Source: CAD feature listing. Evaluate the final solid. Frame: model axes, mm. Coordinates: 2 decimals unless noted, no trailing zeros. Write each loop counter-clockwise with the first axis right and the second up, starting at its lowest first coordinate (ties: lowest second). Pieces come first, ordered by that corner, then holes. Notation, with made-up numbers: M 48.5,44.25 L 55.5,44.25 A17 ccw 55.5,58.25 Z; hole C 25,-16 d7. An arc over 180 degrees is marked long. Write item = value, one per line. Start each with the question number.
1. Pin query (flat end, axial travel): pin 1 Ø3 at (x, y) = (0.9, 15.73) entering from +Z. Return the tip coordinate at first contact, or that it passes through.
2. Section query B-B (z = 0.7). Output: boundary loops of the cut face in (x, y).
3. Section query D-D (x = -33). Output: boundary loops of the cut face in (y, z), then the cut area to 3 significant figures.
4. Section query A-A (y = 0). Output: boundary loops of the cut face in (x, z).
5. Section query C-C (x = 0). Output: boundary loops of the cut face in (y, z).
6. Line query: line 1 along Y through (x, z) = (8, 2.25); line 2 along Y through (x, z) = (-12.5, 1.4); line 3 along X through (y, z) = (6, 1.65). Output: solid intervals per line, ascending.
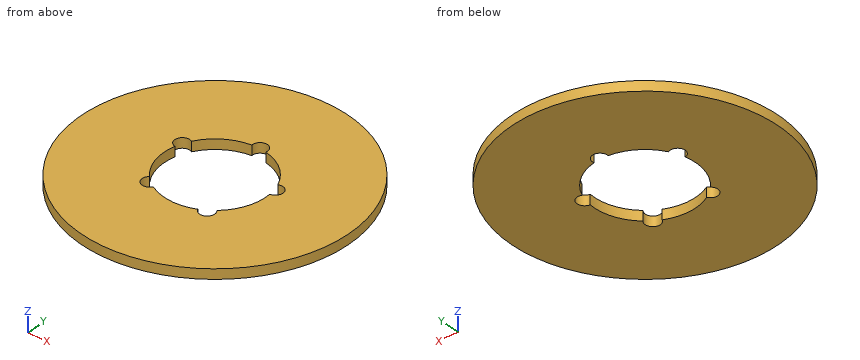
```python
from build123d import *

# Parameters (mm, degrees)
F0_R     = 40.7341209129
F1_DEPTH = 3
F2_R     = 12.35
F3_DEPTH = 5
F4_R     = 15.5
F5_DEPTH = 3
F7_R     = 2.3
F8_DEPTH = 25


# Not quite as in the source:
# - a feature names something its author has since deleted; it is built from what else it names


with BuildPart() as f1:
    # F0 (on Top) → F1 (new body)
    with BuildSketch(Plane.XY):
        Circle(F0_R)
    extrude(amount=F1_DEPTH)

    # F2 (on face) → F3 (cut)
    with BuildSketch(Plane.XY.offset(3)):
        Circle(F2_R)
    extrude(amount=-F3_DEPTH, mode=Mode.SUBTRACT)

    # F4 (on face) → F5 (cut)
    with BuildSketch(Plane.XY.offset(3)):
        Circle(F4_R)
    extrude(amount=-F5_DEPTH, mode=Mode.SUBTRACT)

    # F7 (on face) → F8 (cut)
    with BuildSketch(Plane.XY.offset(3)):
        with Locations((15.2315180749, 3.9969421923)):
            Circle(F7_R)
        with Locations((8.4959734231, -13.2423266768)):
            Circle(F7_R)
        with Locations((-9.9757602438, -12.1809709817)):
            Circle(F7_R)
        with Locations((-14.6723501384, 5.7214666158)):
            Circle(F7_R)
        with Locations((0.8970320341, 15.7257020473)):
            Circle(F7_R)
    extrude(amount=-F8_DEPTH, mode=Mode.SUBTRACT)


solid = f1.part
```
Results are:
q1.pin_1 = through
q2.outline = C 0,0 d81.47; hole M -15.11,3.46 A15.5 ccw -11.47,-10.43 A2.3 ccw long -7.96,-13.3 A15.5 ccw 6.37,-14.13 A2.3 ccw long 10.19,-11.68 A15.5 ccw 15.41,1.7 A2.3 ccw long 14.26,6.08 A15.5 ccw 3.13,15.18 A2.3 ccw long -1.38,15.44 A15.5 ccw -13.46,7.68 A2.3 ccw long Z
q3.outline = M -23.88,0 L 23.88,0 L 23.88,3 L -23.88,3 Z
q3.area = 143 mm^2
q4.outline = M -40.73,0 L -15.5,0 L -15.5,3 L -40.73,3 Z; M 15.5,0 L 40.73,0 L 40.73,3 L 15.5,3 Z
q5.outline = M -40.73,0 L -15.5,0 L -15.5,3 L -40.73,3 Z; M 17.84,0 L 40.73,0 L 40.73,3 L 17.84,3 Z
q6.line_1 = -39.94 to -15.49, 13.28 to 39.94
q6.line_2 = -38.77 to -9.17, 9.17 to 38.77
q6.line_3 = -40.29 to -16.96, 16.36 to 40.29
